from build123d import *

# Parameters (mm, degrees)
ESBO_O2_R                = 1.65
RESSALTO_EXTRUS_O1_DEPTH = 3
CHANFRO1_SIZE            = 4
CHANFRO1_SIZE_2          = 1.865230633
ESBO_O3_W                = 16.82142479
ESBO_O3_H                = 3.834770965
CORTE_EXTRUS_O1_DEPTH    = 5


with BuildPart() as part:
    # Esboço2 → Ressalto-extrusão1 (new body)
    with BuildSketch(Plane.XY):
        with BuildLine():
            Line((15, 2.5), (8.124038405, 2.5))
            ThreePointArc((8.124038405, 2.5), (5.049752469, 6.837397166), (0, 8.5))
            ThreePointArc((0, 8.5), (-6.75, 1.75), (0, -5))
            ThreePointArc((0, -5), (2.5, -4.330127019), (4.330127019, -2.5))
            Line((4.330127019, -2.5), (15, -2.5))
            ThreePointArc((15, -2.5), (17.5, 0), (15, 2.5))
        make_face()
        Circle(ESBO_O2_R, mode=Mode.SUBTRACT)
    extrude(amount=RESSALTO_EXTRUS_O1_DEPTH)

    # Chanfro1
    # the kernel refuses this chamfer: 4, 1.865230633 mm, written as the material it takes off along each edge
    with BuildSketch(Plane(origin=(0, 0, 0), x_dir=(0.6049671971575049, -0.7962503942626293, 0), z_dir=(-0.7962503942626293, -0.6049671971575049, 0))) as chanfro1_piece_1_section:
        Polygon((8.5, CHANFRO1_SIZE), (8.5 - CHANFRO1_SIZE_2, 0), (8.5, 0), align=None)
    chanfro1_piece_1 = revolve(axis=Axis((0, 0, 0), (0, 0, 1)), revolution_arc=142.773518556, mode=Mode.PRIVATE)
    chanfro1_piece_1 = split(chanfro1_piece_1, bisect_by=Plane(origin=(6.168513844, 2.5, 1.415637253), z_dir=(0, 1, 0)), keep=Keep.TOP, mode=Mode.PRIVATE)
    add(chanfro1_piece_1, mode=Mode.SUBTRACT)
    with BuildSketch(Plane(origin=(0, 0, 0), x_dir=(0, -1, 0), z_dir=(-1, 0, 0))) as chanfro1_piece_2_section:
        Polygon((5, CHANFRO1_SIZE), (5 - CHANFRO1_SIZE_2, 0), (5, 0), align=None)
    chanfro1_piece_2 = revolve(axis=Axis((0, 0, 0), (0, 0, 1)), revolution_arc=178.782767485, mode=Mode.PRIVATE)
    chanfro1_piece_2 = split(chanfro1_piece_2, bisect_by=Plane(origin=(1.977914481, -2.5, 1.262439035), z_dir=(0, -1, 0)), keep=Keep.TOP, mode=Mode.PRIVATE)
    add(chanfro1_piece_2, mode=Mode.SUBTRACT)
    with BuildSketch(Plane(origin=(0, 1.75, 0), x_dir=(0, 1, 0), z_dir=(1, 0, 0))) as chanfro1_piece_3:
        Polygon((6.75, CHANFRO1_SIZE), (6.75 - CHANFRO1_SIZE_2, 0), (6.75, 0), align=None)
    revolve(axis=Axis((0, 1.75, 0), (0, 0, 1)), revolution_arc=180, mode=Mode.SUBTRACT)

    # Esboço3 → Corte-extrusão1 (cut)
    with BuildSketch(Plane.XY.offset(3)):
        with Locations((-0.707373788, -4.417385483)):
            Rectangle(ESBO_O3_W, ESBO_O3_H)
    extrude(amount=-CORTE_EXTRUS_O1_DEPTH, mode=Mode.SUBTRACT)


solid = part.part
Model file for the job. Use its own axes, mm. Round coordinates to 2 decimals unless told otherwise and drop trailing zeros. Order: outer loops, then holes, each group sorted by start corner. A loop starts at its lowest first (then second) coordinate and runs counter-clockwise, first axis right, second up. Notation, with made-up numbers: M 58.25,-39.5 L 79.25,-39.5 A28 cw 79.25,-7.5 Z; hole C 86,65.25 d6. An arc over 180 degrees is marked long. Write each question's results on one line, items separated by ' | '. Start each with the question number.
(1) Saw through at B-B, the plane z = 1.9. Give the cut face in (x, y), then the cut area to 3 significant figures.
(2) Probe probe 1 along Y at (x, z) = (13, 1); probe 2 along Y at (x, z) = (-1.25, 2.25); probe 3 along Y at (x, z) = (0.25, 0.9). List the from-to ranges inside material, lowest first. Write a range as from..to.
(3) Saw through at A-A, the plane z = 0.6. Give the cut face in (x, y).
(4) Two-plate mould, pull along X, no slides. Class faces 1 (the face through (17.5, -0.1, 1.5)), 2 (the face through (6, 1, 0)), 3 (the face through (-1.216, 1.115, 1.479)): pulls with the +X half, pulls with the -X half, needs draft (parallel to the pull), parting line crosses it, or undercut.
Established:
1) outline: M -3.9,-2.5 L 15,-2.5 A2.5 ccw 15,2.5 L 7.09,2.5 A7.52 ccw 0,7.52 A5.77 ccw Z; hole C 0,0 d3.3 | area: 150 mm^2
2) probe 1: y = -2.5..2.5 | probe 2: y = -2.5..-1.08, 1.08..7.55 | probe 3: y = -2.5..-1.63, 1.63..7.05
3) outline: M -2.93,-2.5 L 15,-2.5 A2.5 ccw 15,2.5 L 6.45,2.5 A6.91 ccw 0,6.91 A5.16 ccw Z; hole C 0,0 d3.3
4) face 1: pulls with the +X half | face 2: needs draft | face 3: undercut
